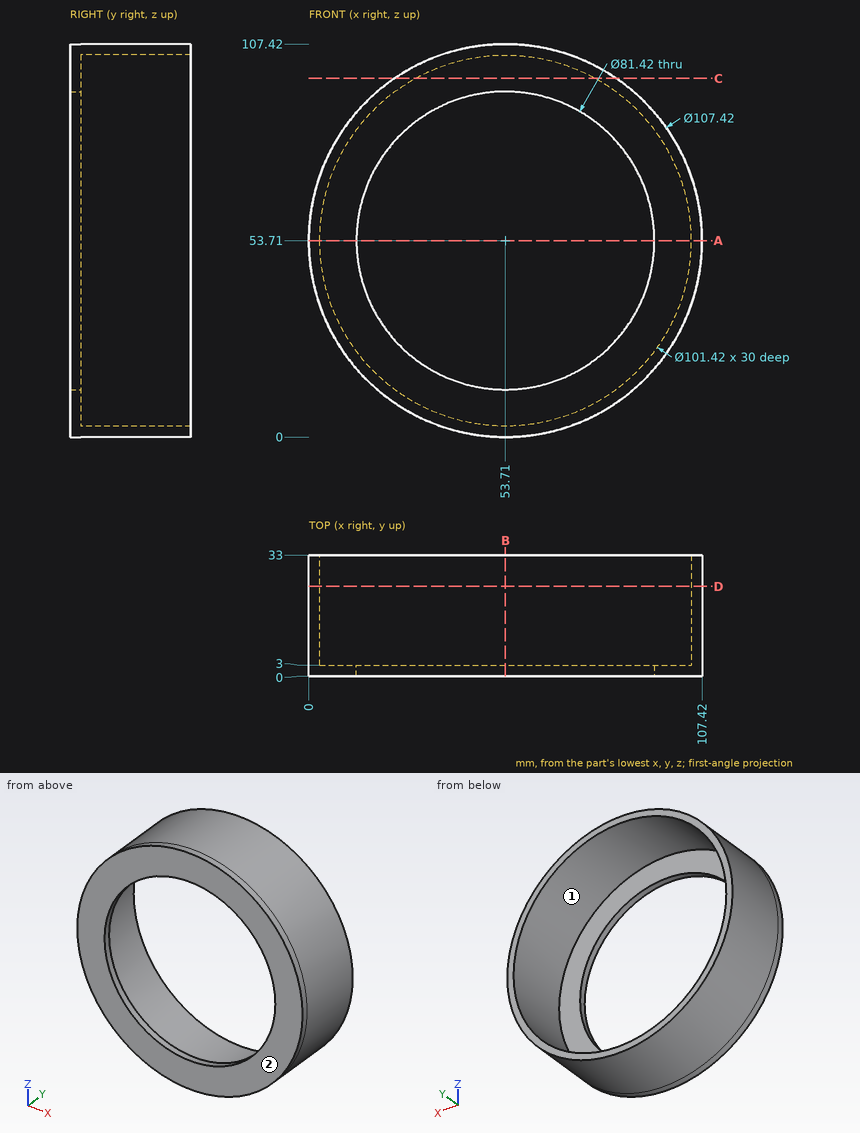
The drawing under review shows one solid part. Ordinate dimensions are in mm from its lowest x, y, z. Round coordinates to 2 decimals unless told otherwise and drop trailing zeros. Loops run counter-clockwise (first coordinate to the right, second up) from the corner with the lowest first, then second, coordinate; pieces in that order, holes last. Notation, with made-up numbers: M 64.25,10 L 101.25,10 A6 cw 101.25,14 Z; hole C 71.25,9.25 d2. An arc over 180 degrees is marked long. Answer as CSV lines item,"result". Start each with the question number.
Item 1: Mouldability with a two-part tool opening along Z and no side actions: class the marked faces 1 and 2 as released by +Z, released by -Z, zero draft, split by the parting line, or undercut.
Item 2: Consider section D-D (y = 24.5). Write out the cut boundary in (x, z).
Item 3: Consider section C-C (z = 98). Write out the cut boundary in (x, y), then the cut area to 3 significant figures.
Item 4: Insertion check: P1, Ø1.5, axis at y = 4.5, z = 11, coming from the +X side; P2, Ø3, axis at x = 84.5, y = 27, coming from the -Z side; P3, Ø5, axis at y = 5, z = 47.5, coming from the +X side; P4, Ø4, axis at x = 13.5, z = 31.5, coming from the -Y side. Each pin has a flat end and moves straight along its axis. Give the tip position at first contact, or say it passes through.
Item 5: Consider section B-B (x = 53.71). Write out the cut boundary in (y, z).
Item 6: Wall thickness on line 1 (Z direction, x = 53.71, y = 1.2); line 2 (X direction, y = 2, z = 53); line 3 (Z direction, x = 53.71, y = 11.75): over which ranges is each line inside the solid? List them lowest first. Write a range as [from, to].
Item 7: Consider section A-A (z = 53.71). Write out the cut boundary in (x, y).
Answer:
1,face 1,"undercut"
1,face 2,"zero draft"
2,outline,"C 53.71,53.71 d107.42; hole C 53.71,53.71 d101.42"
3,outline,"M 23.33,0 L 84.09,0 L 84.09,33 L 78.41,33 L 78.41,3 L 29.01,3 L 29.01,33 L 23.33,33 Z"
3,area,"524 mm^2"
4,P1,"stops at x = 87.24"
4,P2,"stops at z = 8.69"
4,P3,"stops at x = 107.29"
4,P4,"stops at y = 0"
5,outline,"M 0,0 L 33,0 L 33,3 L 3,3 L 3,13 L 0,13 Z; M 0,94.42 L 3,94.42 L 3,104.42 L 33,104.42 L 33,107.42 L 0,107.42 Z"
6,line 1,"z = [0, 13], [94.42, 107.42]"
6,line 2,"x = [0, 13.01], [94.41, 107.42]"
6,line 3,"z = [0, 3], [104.42, 107.42]"
7,outline,"M 0,0 L 13,0 L 13,3 L 3,3 L 3,33 L 0,33 Z; M 94.42,0 L 107.42,0 L 107.42,33 L 104.42,33 L 104.42,3 L 94.42,3 Z"
